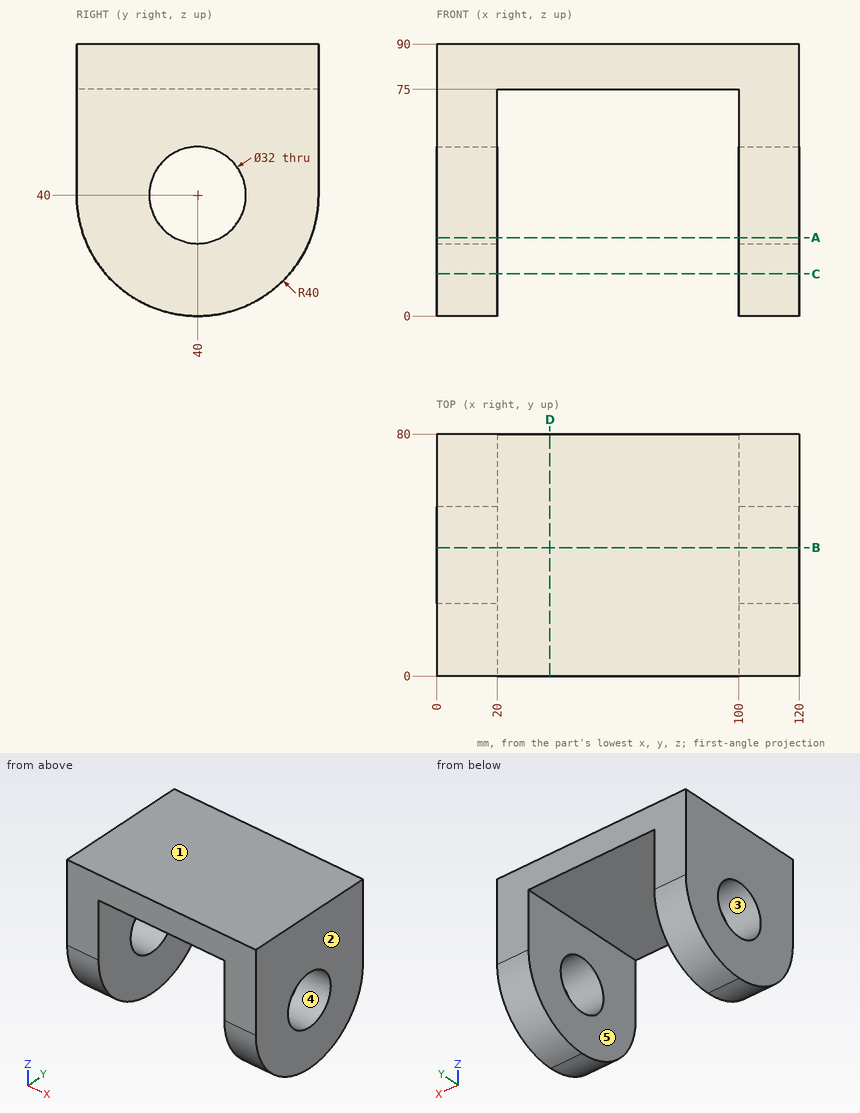
Geometry check sheet. Reference: drawing and pictorial views, mm from the part's lowest x, y, z. A direction names the side the tool comes from. Round coordinates to 2 decimals unless told otherwise and drop trailing zeros. Loops run counter-clockwise (first coordinate to the right, second up) from the corner with the lowest first, then second, coordinate; pieces in that order, holes last. Notation, with made-up numbers: (-10.75, 15.25) - (19.25, 15.25) arc R23 cw to (19.25, 45.25) - close; hole circle Ø4 at (-20, 11.25). An arc over 180 degrees is marked (long way). Write item = value, one per line. Start each with the question number.
Q1. Depth check by flat-ended pin: P1, Ø24, axis at x = 43.5, y = 31, coming from the -Z side. Enter the tip coordinate at first touch or a pass-through.
Q2. Thickness scan on L1, parallel to Z at x = 106, y = 40; L2, parallel to X at y = 10, z = 29; L3, parallel to Z at x = 50.5, y = 65. Record the ranges inside material, lowest first.
Q3. Release check for a two-part mould opening along Z. For the marked faces 1, 2 and 3 record: pulls with the +Z half, pulls with the -Z half, needs draft (parallel to the pull), parting line crosses it, or undercut.
Q4. Section check C-C (z = 14). Record the boundary of the cut face in (x, y).
Q5. Access from +Z, -Z, +X, -X, +Y, -Y to the whole of each face (thin tool, end or side, straight path). Record for the marked faces 4 and 5.
Q6. Section check A-A (z = 26). Record the boundary of the cut face in (x, y).
Q7. Section check D-D (x = 37.5). Record the boundary of the cut face in (y, z), plus the area to 3 significant figures.
Q8. Section check B-B (y = 42.5). Record the boundary of the cut face in (x, z), plus the area to 3 significant figures.
Derived:
q1.P1 = 75
q2.L1 = 0 to 24, 56 to 90
q2.L2 = 0 to 20, 100 to 120
q2.L3 = 75 to 90
q3.face_1 = pulls with the +Z half
q3.face_2 = needs draft
q3.face_3 = undercut
q4.outline = (0, 9.6) - (20, 9.6) - (20, 70.4) - (0, 70.4) - close; (100, 9.6) - (120, 9.6) - (120, 70.4) - (100, 70.4) - close
q5.face_4 = +X, -X
q5.face_5 = -Z, +Y, -Y
q6.outline = (0, 2.53) - (20, 2.53) - (20, 32.25) - (0, 32.25) - close; (0, 47.75) - (20, 47.75) - (20, 77.47) - (0, 77.47) - close; (100, 2.53) - (120, 2.53) - (120, 32.25) - (100, 32.25) - close; (100, 47.75) - (120, 47.75) - (120, 77.47) - (100, 77.47) - close
q7.outline = (0, 75) - (80, 75) - (80, 90) - (0, 90) - close
q7.area = 1,200 mm^2
q8.outline = (0, 0.08) - (20, 0.08) - (20, 24.2) - (0, 24.2) - close; (0, 55.8) - (20, 55.8) - (20, 75) - (100, 75) - (100, 55.8) - (120, 55.8) - (120, 90) - (0, 90) - close; (100, 0.08) - (120, 0.08) - (120, 24.2) - (100, 24.2) - close
q8.area = 3,530 mm^2
